Design review of the part built by this model. Coordinates are the model's own, in mm. A direction names the side the tool comes from. Coordinates: 2 decimals unless noted, no trailing zeros. Write each loop counter-clockwise with the first axis right and the second up, starting at its lowest first coordinate (ties: lowest second). Pieces come first, ordered by that corner, then holes. Notation, with made-up numbers: (24, 42) -> (71, 42) arc R16 cw to (71, 72) -> close; hole circle Ø1 at (43, 47). An arc over 180 degrees is marked (long way). One line per question, with ' | ' between items. Start each with the question number.
Q1. For P1, Ø3.5, axis at y = 8.89, z = 7.62, coming from the +X side; P2, Ø1, axis at y = 2.5, z = 18, coming from the -X side; P3, Ø4, axis at y = 2.5, z = 18.5, coming from the -X side, all flat-tipped, find the tip position at first contact; note any pin that passes through.
Q2. Draft analysis for pull direction Y (two halves, no side actions). For faces 1 (the flat face through (0, 0, 25.4)), 2 (the flat face through (-1, 16.292, 13)), 3 (the cylindrical face through (15.73, 12.06, 6.31)), state which applies: pulls with the +Y half, pulls with the -Y half, needs draft (parallel to the pull), parting line crosses it, or undercut.
Q3. Add section B-B on x = 4. State the section outline as (y, z) points, and give its area (3 significant figures).
Q4. Add section C-C on y = -8.89. State the section outline as (x, z) points.
Q5. Add section D-D on z = 3.75. State the section outline as (x, y) points, and give its area (3 significant figures).
Q6. For faces 4 (the flat face through (0, 0, 0)), 5 (the flat face through (13.614, -10, 17)), list the 3-axis set-ups (+Z, -Z, +X, -X, +Y, -Y) from which the entire face can be reached by the end or side of a thin tool; tool diameter is ignored.
Q7. Wall thickness on probe 1 along Z at (x, y) = (-1.5, 8.89); probe 2 along Z at (x, y) = (-9, 8); probe 3 along Y at (x, z) = (8, 17): over which ranges is each line inside the solid? List them lowest first.
Q8. Add section A-A on z = 17.78. State the section outline as (x, y) points, and give its area (3 significant figures).
from build123d import *

# Parameters (mm, degrees)
F1_DEPTH       = 25.4
F3_D           = 2.0828
F3_CBORE_D     = 6.858
F3_CBORE_DEPTH = 4.1656
F5_D           = 2.0828


with BuildPart() as f1:
    # F0 (on Top) → F1 (new body)
    with BuildSketch(Plane.XY):
        with BuildLine():
            Line((-17.78, -6.35), (-17.78, -16.29156))
            Line((-17.78, -16.29156), (15.24, -16.29156))
            ThreePointArc((15.24, -16.29156), (17.036051, -15.547611), (17.78, -13.75156))
            Line((17.78, -13.75156), (17.78, 13.75156))
            ThreePointArc((17.78, 13.75156), (17.036051, 15.547611), (15.24, 16.29156))
            Line((15.24, 16.29156), (-17.78, 16.29156))
            Line((-17.78, 16.29156), (-17.78, 6.35))
            ThreePointArc((-17.78, 6.35), (-11.43, 0), (-17.78, -6.35))
        make_face()
    extrude(amount=F1_DEPTH)

    # F3 (through all)
    with Locations(Plane.YZ.offset(17.78)):
        with Locations((-8.89, 17.78), (-8.89, 7.62), (8.89, 17.78), (8.89, 7.62)):
            CounterBoreHole(F3_D / 2, F3_CBORE_D / 2, F3_CBORE_DEPTH)

    # F5 (through all)
    with Locations(Plane(origin=(0, 0, 0), x_dir=(1, 0, 0), z_dir=(0, 0, -1))):
        with Locations((0, 5.08), (0, -5.08)):
            Hole(F5_D / 2)


solid = f1.part
Output values:
1) P1: stops at x = 13.61 | P2: stops at x = -12.18 | P3: stops at x = -13.3
2) face 1: needs draft | face 2: pulls with the +Y half | face 3: undercut
3) outline: (-16.29, 0) -> (16.29, 0) -> (16.29, 25.4) -> (-16.29, 25.4) -> close; hole circle Ø2.08 at (-8.89, 7.62); hole circle Ø2.08 at (-8.89, 17.78); hole circle Ø2.08 at (8.89, 7.62); hole circle Ø2.08 at (8.89, 17.78) | area: 814 mm2
4) outline: (-17.78, 0) -> (17.78, 0) -> (17.78, 4.19) -> (13.61, 4.19) -> (13.61, 6.58) -> (-17.78, 6.58) -> close; (-17.78, 8.66) -> (13.61, 8.66) -> (13.61, 11.05) -> (17.78, 11.05) -> (17.78, 14.35) -> (13.61, 14.35) -> (13.61, 16.74) -> (-17.78, 16.74) -> close; (-17.78, 18.82) -> (13.61, 18.82) -> (13.61, 21.21) -> (17.78, 21.21) -> (17.78, 25.4) -> (-17.78, 25.4) -> close
5) outline: (-17.78, -16.29) -> (15.24, -16.29) arc R2.54 ccw to (17.78, -13.75) -> (17.78, 13.75) arc R2.54 ccw to (15.24, 16.29) -> (-17.78, 16.29) -> (-17.78, 6.35) arc R6.35 cw to (-17.78, -6.35) -> close; hole circle Ø2.08 at (0, -5.08); hole circle Ø2.08 at (0, 5.08) | area: 1,090 mm2
6) face 4: -Z, +X, -X, +Y, -Y | face 5: +X
7) probe 1: z = 0 to 6.58, 8.66 to 16.74, 18.82 to 25.4 | probe 2: z = 0 to 7.08, 8.16 to 17.24, 18.32 to 25.4 | probe 3: y = -16.29 to -9.58, -8.2 to 8.2, 9.58 to 16.29
8) outline: (-17.78, -16.29) -> (15.24, -16.29) arc R2.54 ccw to (17.78, -13.75) -> (17.78, -12.32) -> (13.61, -12.32) -> (13.61, -9.93) -> (-17.78, -9.93) -> close; (-17.78, -7.85) -> (13.61, -7.85) -> (13.61, -5.46) -> (17.78, -5.46) -> (17.78, 5.46) -> (13.61, 5.46) -> (13.61, 7.85) -> (-17.78, 7.85) -> (-17.78, 6.35) arc R6.35 cw to (-17.78, -6.35) -> close; (-17.78, 9.93) -> (13.61, 9.93) -> (13.61, 12.32) -> (17.78, 12.32) -> (17.78, 13.75) arc R2.54 ccw to (15.24, 16.29) -> (-17.78, 16.29) -> close; hole circle Ø2.08 at (0, -5.08); hole circle Ø2.08 at (0, 5.08) | area: 898 mm2
